Build history of the part. All positions in model axes, mm. Face numbers are marked on the shaded views. A direction names the side the tool comes from. Round coordinates to 2 decimals unless told otherwise and drop trailing zeros. Loops run counter-clockwise (first coordinate to the right, second up) from the corner with the lowest first, then second, coordinate; pieces in that order, holes last. Notation, with made-up numbers: (-13.5, 78) - (21.5, 78) arc R26 ccw to (21.5, 99) - close; hole circle Ø4 at (-0.5, 0.25). An arc over 180 degrees is marked (long way). Put each result on its own line as item: value. Start each with the question number.
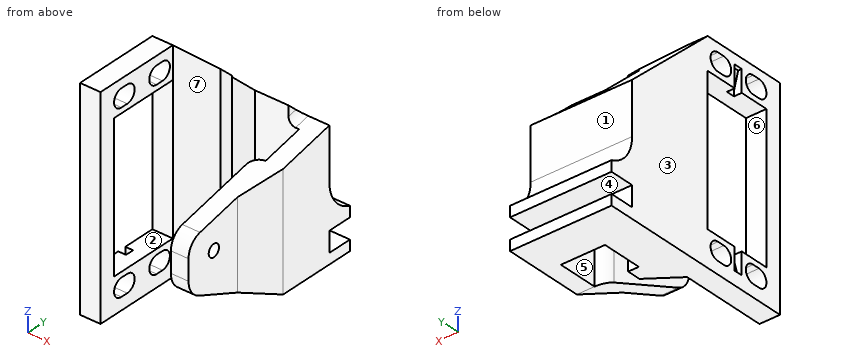
from build123d import *

# Parameters (mm, degrees)
BOSS_EXTRUDE1_DEPTH     = 60
CUT_EXTRUDE1_REACH      = 252.16
SKETCH4_W               = 41
SKETCH4_H               = 20
CUT_EXTRUDE2_DEPTH      = 1
CUT_EXTRUDE2_DEPTH_BACK = 1.4
CUT_EXTRUDE2_START      = -14
SKETCH2_R               = 1.75
CUT_EXTRUDE3_DEPTH      = 5
SKETCH6_W               = 3
SKETCH6_H               = 7
BOSS_EXTRUDE2_DEPTH     = 28.75
FILLET1_R               = 10
CUT_EXTRUDE4_REACH      = 252.16
CUT_EXTRUDE5_REACH      = 252.16
CUT_EXTRUDE6_REACH      = 252.16
FILLET2_R               = 5
FILLET3_R               = 6
FILLET4_R               = 2


with BuildPart() as part:
    # Sketch1 → Boss-Extrude1 (new body)
    with BuildSketch(Plane.XY):
        with BuildLine():
            Line((391.716436469, -195.128416651), (404.216436469, -195.128416651))
            Line((404.216436469, -195.128416651), (404.216436469, -206.578416651))
            ThreePointArc((404.216436469, -206.578416651), (402.095116126, -207.457096307), (401.216436469, -209.578416651))
            Line((401.216436469, -209.578416651), (401.216436469, -235.169373092))
            Line((401.216436469, -235.169373092), (406.216436469, -235.169373092))
            Line((406.216436469, -235.169373092), (406.216436469, -218.547748038))
            Line((406.216436469, -218.547748038), (409.216436469, -206.578416651))
            Line((409.216436469, -206.578416651), (409.216436469, -190.835999092))
            Line((409.216436469, -190.835999092), (380.466436469, -190.835999092))
            Line((380.466436469, -190.835999092), (380.466436469, -241.150690411))
            Line((380.466436469, -241.150690411), (386.266436469, -241.150690411))
            Line((386.266436469, -241.150690411), (386.266436469, -216.54774804))
            Line((386.266436469, -216.54774804), (394.716436469, -210.46208716))
            Line((394.716436469, -210.46208716), (394.716436469, -206.628416651))
            Line((394.716436469, -206.628416651), (391.716436469, -206.628416651))
            Line((391.716436469, -206.628416651), (391.716436469, -195.128416651))
        make_face()
    extrude(amount=BOSS_EXTRUDE1_DEPTH)

    # Cut-Extrude1: up to this face of the body (flat: up to its plane)
    cut_extrude1_end = Plane(part.part.faces().sort_by_distance((386.266436469, -228.849219226, 30))[0])
    # Sketch4 → Cut-Extrude1 (cut, up to the picked face)
    with BuildSketch(Plane.ZY.offset(-380.466436469), mode=Mode.PRIVATE) as cut_extrude1_sk1:
        with BuildLine():
            Line((57.5, -232.04774804), (57.5, -234.04774804))
            ThreePointArc((57.5, -234.04774804), (55, -236.54774804), (52.5, -234.04774804))
            Line((52.5, -234.04774804), (52.5, -232.04774804))
            ThreePointArc((52.5, -232.04774804), (55, -229.54774804), (57.5, -232.04774804))
        make_face()
    cut_extrude1_tool1 = split(extrude(cut_extrude1_sk1.sketch, amount=-CUT_EXTRUDE1_REACH, mode=Mode.PRIVATE), bisect_by=cut_extrude1_end, keep=Keep.BOTH, mode=Mode.PRIVATE)
    # Sketch4 → Cut-Extrude1 (cut, up to the picked face)
    with BuildSketch(Plane.ZY.offset(-380.466436469), mode=Mode.PRIVATE) as cut_extrude1_sk2:
        with Locations((30.5, -226.54774804)):
            Rectangle(SKETCH4_W, SKETCH4_H)
    cut_extrude1_tool2 = split(extrude(cut_extrude1_sk2.sketch, amount=-CUT_EXTRUDE1_REACH, mode=Mode.PRIVATE), bisect_by=cut_extrude1_end, keep=Keep.BOTH, mode=Mode.PRIVATE)
    # Sketch4 → Cut-Extrude1 (cut, up to the picked face)
    with BuildSketch(Plane.ZY.offset(-380.466436469), mode=Mode.PRIVATE) as cut_extrude1_sk3:
        with BuildLine():
            Line((8.5, -222.04774804), (8.5, -220.04774804))
            ThreePointArc((8.5, -220.04774804), (6, -217.54774804), (3.5, -220.04774804))
            Line((3.5, -220.04774804), (3.5, -222.04774804))
            ThreePointArc((3.5, -222.04774804), (6, -224.54774804), (8.5, -222.04774804))
        make_face()
    cut_extrude1_tool3 = split(extrude(cut_extrude1_sk3.sketch, amount=-CUT_EXTRUDE1_REACH, mode=Mode.PRIVATE), bisect_by=cut_extrude1_end, keep=Keep.BOTH, mode=Mode.PRIVATE)
    # Sketch4 → Cut-Extrude1 (cut, up to the picked face)
    with BuildSketch(Plane.ZY.offset(-380.466436469), mode=Mode.PRIVATE) as cut_extrude1_sk4:
        with BuildLine():
            Line((3.5, -232.04774804), (3.5, -234.04774804))
            ThreePointArc((3.5, -234.04774804), (6, -236.54774804), (8.5, -234.04774804))
            Line((8.5, -234.04774804), (8.5, -232.04774804))
            ThreePointArc((8.5, -232.04774804), (6, -229.54774804), (3.5, -232.04774804))
        make_face()
    cut_extrude1_tool4 = split(extrude(cut_extrude1_sk4.sketch, amount=-CUT_EXTRUDE1_REACH, mode=Mode.PRIVATE), bisect_by=cut_extrude1_end, keep=Keep.BOTH, mode=Mode.PRIVATE)
    # Sketch4 → Cut-Extrude1 (cut, up to the picked face)
    with BuildSketch(Plane.ZY.offset(-380.466436469), mode=Mode.PRIVATE) as cut_extrude1_sk5:
        with BuildLine():
            Line((57.5, -220.04774804), (57.5, -222.04774804))
            ThreePointArc((57.5, -222.04774804), (55, -224.54774804), (52.5, -222.04774804))
            Line((52.5, -222.04774804), (52.5, -220.04774804))
            ThreePointArc((52.5, -220.04774804), (55, -217.54774804), (57.5, -220.04774804))
        make_face()
    cut_extrude1_tool5 = split(extrude(cut_extrude1_sk5.sketch, amount=-CUT_EXTRUDE1_REACH, mode=Mode.PRIVATE), bisect_by=cut_extrude1_end, keep=Keep.BOTH, mode=Mode.PRIVATE)
    add(cut_extrude1_tool1.solids().sort_by(Axis((380.466436, -233.047748, 55), (1, 0, 0)))[0], mode=Mode.SUBTRACT)
    add(cut_extrude1_tool2.solids().sort_by(Axis((380.466436, -226.547748, 30.5), (1, 0, 0)))[0], mode=Mode.SUBTRACT)
    add(cut_extrude1_tool3.solids().sort_by(Axis((380.466436, -221.047748, 6), (1, 0, 0)))[0], mode=Mode.SUBTRACT)
    add(cut_extrude1_tool4.solids().sort_by(Axis((380.466436, -233.047748, 6), (1, 0, 0)))[0], mode=Mode.SUBTRACT)
    add(cut_extrude1_tool5.solids().sort_by(Axis((380.466436, -221.047748, 55), (1, 0, 0)))[0], mode=Mode.SUBTRACT)

    # Sketch5 → Cut-Extrude2 (cut, two sides: drawn at the far end of the back side and taken through both)
    with BuildSketch(Plane.XZ.offset(241.150690411).offset(CUT_EXTRUDE2_START - CUT_EXTRUDE2_DEPTH_BACK)):
        Polygon((380.466436469, 51), (382.666436469, 51), (382.666436469, 52.5), (381.466436469, 57.2), (380.466436469, 57.2), align=None)
        Polygon((380.466436469, 10), (382.666436469, 10), (382.666436469, 8.5), (381.466436469, 3.8), (380.466436469, 3.8), align=None)
    extrude(amount=CUT_EXTRUDE2_DEPTH + CUT_EXTRUDE2_DEPTH_BACK, mode=Mode.SUBTRACT)

    # Sketch2 → Cut-Extrude3 (cut)
    with BuildSketch(Plane(origin=(406.216436469, 0, 0), x_dir=(0, 0, -1), z_dir=(1, 0, 0))):
        with Locations((-20, -226.54774804)):
            Circle(SKETCH2_R)
    extrude(amount=-CUT_EXTRUDE3_DEPTH, mode=Mode.SUBTRACT)

    # Sketch6 → Boss-Extrude2 (add)
    with BuildSketch(Plane(origin=(409.216436469, 0, 0), x_dir=(0, 0, -1), z_dir=(1, 0, 0))):
        with Locations((-1.5, -187.335999092)):
            Rectangle(SKETCH6_W, SKETCH6_H)
        with Locations((-10.25, -187.335999092)):
            Rectangle(SKETCH6_W, SKETCH6_H)
    extrude(amount=-BOSS_EXTRUDE2_DEPTH)

    # Fillet1
    # the kernel refuses this fillet: 10 mm, written as the material it adds along each edge
    with BuildSketch(Plane(origin=(409.216436469, -190.835999092, 11.75), x_dir=(0, 1, 0), z_dir=(-1, 0, 0))) as fillet1_piece_1:
        with BuildLine():
            CenterArc((10, -9.539392014), FILLET1_R, 107.457603124, 72.542396876)
            Line((0, -9.539392014), (-0.2, -9.539392014))
            Line((-0.2, -9.539392014), (-0.2, 0))
            Line((-0.2, 0), (0, 0.2))
            ThreePointArc((0, 0.2), (3.5, 0.2), (6.94, 0.19078784))
            Line((6.94, 0.19078784), (7, 0))
        make_face()
    extrude(amount=28.75)

    # Cut-Extrude4: up to this face of the body (flat: up to its plane)
    cut_extrude4_end = Plane(part.part.faces().sort_by_distance((409.216436469, -198.059355839, 28.706804471))[0])
    # Sketch7 → Cut-Extrude4 (cut, up to the picked face)
    with BuildSketch(Plane.ZY.offset(-380.466436469), mode=Mode.PRIVATE) as cut_extrude4_sk1:
        Polygon((60, -190.835999092), (36, -190.835999092), (60, -216.54774804), align=None)
    cut_extrude4_tool1 = split(extrude(cut_extrude4_sk1.sketch, amount=-CUT_EXTRUDE4_REACH, mode=Mode.PRIVATE), bisect_by=cut_extrude4_end, keep=Keep.BOTH, mode=Mode.PRIVATE)
    add(cut_extrude4_tool1.solids().sort_by(Axis((380.466436, -199.406582, 52), (1, 0, 0)))[0], mode=Mode.SUBTRACT)

    # Cut-Extrude5: up to this face of the body (flat: up to its plane)
    cut_extrude5_end = Plane(part.part.faces().sort_by_distance((401.216436469, -222.505111575, 29.644283509))[0])
    # Sketch8 → Cut-Extrude5 (cut, up to the picked face)
    with BuildSketch(Plane(origin=(409.216436469, 0, 0), x_dir=(0, 0, -1), z_dir=(1, 0, 0)), mode=Mode.PRIVATE) as cut_extrude5_sk1:
        Polygon((-36, -235.169373092), (-60, -235.169373092), (-60, -190.835999092), (-36, -190.835999092), (-26.135796826, -235.169373092), align=None)
    cut_extrude5_tool1 = split(extrude(cut_extrude5_sk1.sketch, amount=-CUT_EXTRUDE5_REACH, mode=Mode.PRIVATE), bisect_by=cut_extrude5_end, keep=Keep.BOTH, mode=Mode.PRIVATE)
    add(cut_extrude5_tool1.solids().sort_by(Axis((409.216436, -214.262283, 45.393819), (-1, 0, 0)))[0], mode=Mode.SUBTRACT)

    # Cut-Extrude6: up to this face of the body (flat: up to its plane)
    cut_extrude6_end = Plane(part.part.faces().sort_by_distance((401.216436469, -221.894565092, 14.466227032))[0])
    # Sketch10 → Cut-Extrude6 (cut, up to the picked face)
    with BuildSketch(Plane(origin=(409.216436469, 0, 0), x_dir=(0, 0, -1), z_dir=(1, 0, 0)), mode=Mode.PRIVATE) as cut_extrude6_sk1:
        Polygon((0, -206.578416651), (0, -242.75353584), (-15.622362106, -242.75353584), align=None)
    cut_extrude6_tool1 = split(extrude(cut_extrude6_sk1.sketch, amount=-CUT_EXTRUDE6_REACH, mode=Mode.PRIVATE), bisect_by=cut_extrude6_end, keep=Keep.BOTH, mode=Mode.PRIVATE)
    add(cut_extrude6_tool1.solids().sort_by(Axis((409.216436, -230.695163, 5.207454), (-1, 0, 0)))[0], mode=Mode.SUBTRACT)

    # Fillet2
    fillet2_edges = [part.edges().sort_by_distance(p)[0] for p in [
        (403.716436469, -235.169373092, 26.135796826),
    ]]
    fillet(fillet2_edges, radius=FILLET2_R)

    # Fillet3
    fillet3_edges = [part.edges().sort_by_distance(p)[0] for p in [
        (403.716436469, -235.169373092, 12.347112725),
    ]]
    fillet(fillet3_edges, radius=FILLET3_R)

    # Fillet4
    fillet4_edges = [part.edges().sort_by_distance(p)[0] for p in [
        (401.216436469, -192.982207872, 35.522467217),
    ]]
    fillet(fillet4_edges, radius=FILLET4_R)


solid = part.part
1) Slice it at C-C, the plane z = 45. Write the cut outline in (x, y), and give its area (3 significant figures).
2) Which spindle directions (+Z, -Z, +X, -X, +Y, -Y) get a long thin tool onto all of the face, cutting with end or side? Do the marked faces 4, 5, 6 and 7. Say none if no direction does.
3) Slice it at D-D, the plane z = 20. Write the cut outline in (x, y), and give its area (3 significant figures).
4) Pull direction Y, two halves, no side cores. Call the marked faces 1, 2 and 3: pulls with the +Y half, pulls with the -Y half, needs draft (parallel to the pull), parting line crosses it, or undercut.
5) Drop flat-ended pins along their axis: pin 1 Ø13 at (y, z) = (-221, 22.5) entering from -X; pin 2 Ø8.5 at (y, z) = (-229.5, 13.5) entering from +X; pin 3 Ø1.8 at (x, z) = (381, 55.5) entering from +Y; pin 4 Ø6 at (x, z) = (389, 48.5) entering from +Y. Give the stop position or say it passes through.
6) Slice it at A-A, the plane x = 385.5. State how many separate pieces and enclosed holes the cut face has, and give its area (3 significant figures).
7) Slice it at B-B, the plane y = -198.5. Write the cut outline in (x, z), and give its area (3 significant figures).
8) Drill centre lines: line 1 (X direction, y = -202.5, z = 26); line 2 (Y direction, x = 404.05, z = 20); line 3 (Y direction, x = 398, z = 7). Where is each one in solid material? Low to high. Write a range as [from, to].
Taken from the geometry:
1. outline: (380.47, -241.15) - (386.27, -241.15) - (386.27, -236.55) - (380.47, -236.55) - close; (380.47, -216.55) - (386.27, -216.55) - (394.72, -210.46) - (394.72, -206.63) - (391.72, -206.63) - (391.72, -200.48) - (380.47, -200.48) - close
1. area: 212 mm2
2. face 4: +X, -X, +Y
2. face 5: +Z, -Z
2. face 6: +X, -X
2. face 7: +Z, -Z, -Y
3. outline: (380.47, -241.15) - (386.27, -241.15) - (386.27, -236.55) - (380.47, -236.55) - close; (380.47, -216.55) - (386.27, -216.55) - (394.72, -210.46) - (394.72, -206.63) - (391.72, -206.63) - (391.72, -195.13) - (404.22, -195.13) - (404.22, -206.58) arc R3 ccw to (401.22, -209.58) - (401.22, -224.8) - (406.22, -224.8) - (406.22, -218.55) - (409.22, -206.58) - (409.22, -190.75) - (380.47, -190.75) - close; (401.22, -235.17) - (406.22, -235.17) - (406.22, -228.3) - (401.22, -228.3) - close
3. area: 596 mm2
4. face 1: pulls with the +Y half
4. face 2: undercut
4. face 3: needs draft
5. pin 1: stops at x = 380.47
5. pin 2: stops at x = 406.22
5. pin 3: stops at y = -210.76
5. pin 4: stops at y = -201.01
6. separate pieces: 1
6. enclosed holes: 5
6. area: 1,830 mm2
7. outline: (380.47, 0) - (391.72, 0) - (391.72, 43.15) - (380.47, 43.15) - close; (404.22, 0) - (409.22, 0) - (409.22, 34.29) - (404.22, 34.29) - close
7. area: 657 mm2
8. line 1: x = [380.47, 391.72], [404.22, 409.22]
8. line 2: y = [-235.17, -228.3], [-224.8, -206.58], [-195.13, -190.75]
8. line 3: y = [-195.13, -190.84]
